Build history of the part. All positions in model axes, mm. Face numbers are marked on the shaded views. Round coordinates to 2 decimals unless told otherwise and drop trailing zeros. Loops run counter-clockwise (first coordinate to the right, second up) from the corner with the lowest first, then second, coordinate; pieces in that order, holes last. Notation, with made-up numbers: (89, -30) - (137, -30) arc R25 ccw to (137, -7) - close; hole circle Ø4 at (-35.75, 56). An arc over 180 degrees is marked (long way). Put each result on its own line as item: value. Start each with the question number.
from build123d import *

# Parameters (mm, degrees)
SKETCH2_W                                       = 20
SKETCH2_H                                       = 44
BOSS_EXTRUDE2_DEPTH                             = 0.5
SKETCH4_R                                       = 3.5
BOSS_EXTRUDE3_DEPTH                             = 8
CSK_FOR_M3_FLAT_HEAD_MACHINE_SCREW1_D           = 3.2
CSK_FOR_M3_FLAT_HEAD_MACHINE_SCREW1_DEPTH       = 13.03862301
CSK_FOR_M3_FLAT_HEAD_MACHINE_SCREW1_CSINK_D     = 6.3
CSK_FOR_M3_FLAT_HEAD_MACHINE_SCREW1_CSINK_ANGLE = 90
CSK_FOR_M3_FLAT_HEAD_MACHINE_SCREW1_TIP         = 0.96137699


with BuildPart() as part:
    # Sketch2 → Boss-Extrude2 (new body)
    with BuildSketch(Plane(origin=(0, 0, 0), x_dir=(1, 0, 0), z_dir=(0, 1, 0))):
        with Locations((10, 22)):
            Rectangle(SKETCH2_W, SKETCH2_H)
    extrude(amount=BOSS_EXTRUDE2_DEPTH)

    # Sketch4 → Boss-Extrude3 (add)
    with BuildSketch(Plane(origin=(0, 0, 0), x_dir=(1, 0, 0), z_dir=(0, 1, 0))):
        with Locations(Location((20, 44, 0), (0, 0, 270))):
            Circle(SKETCH4_R)
        with Locations(Location((0, 44, 0), (0, 0, 90))):
            Circle(SKETCH4_R)
        with Locations(Location((20, 0, 0), (0, 0, 90))):
            Circle(SKETCH4_R)
        with Locations(Location((0, 0, 0), (0, 0, 90))):
            Circle(SKETCH4_R)
    extrude(amount=BOSS_EXTRUDE3_DEPTH)

    # CSK for M3 Flat Head Machine Screw1
    with Locations(Plane(origin=(0, 8, 0), x_dir=(1, 0, 0), z_dir=(0, 1, 0))):
        with Locations((20, 44), (0, 44), (0, 0), (20, 0)):
            CounterSinkHole(CSK_FOR_M3_FLAT_HEAD_MACHINE_SCREW1_D / 2, CSK_FOR_M3_FLAT_HEAD_MACHINE_SCREW1_CSINK_D / 2, depth=CSK_FOR_M3_FLAT_HEAD_MACHINE_SCREW1_DEPTH, counter_sink_angle=CSK_FOR_M3_FLAT_HEAD_MACHINE_SCREW1_CSINK_ANGLE)
            with Locations((0, 0, -(CSK_FOR_M3_FLAT_HEAD_MACHINE_SCREW1_DEPTH + CSK_FOR_M3_FLAT_HEAD_MACHINE_SCREW1_TIP / 2))):  # 118° drill point
                Cone(0, CSK_FOR_M3_FLAT_HEAD_MACHINE_SCREW1_D / 2, CSK_FOR_M3_FLAT_HEAD_MACHINE_SCREW1_TIP, mode=Mode.SUBTRACT)


solid = part.part
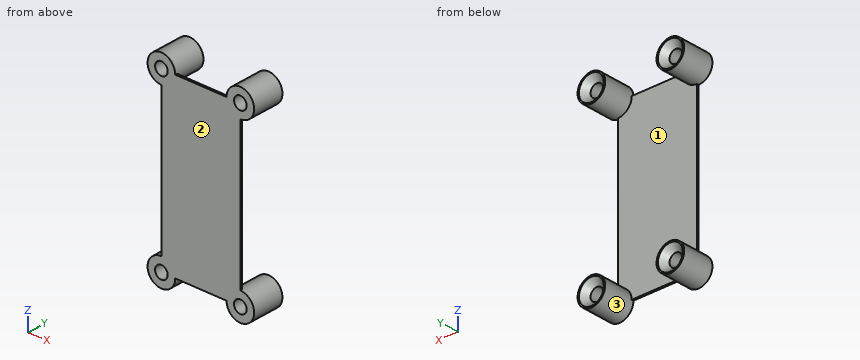
Item 1: Drop flat-ended pins along their axis: pin 1 Ø1.9 at (x, z) = (0, -44) entering from -Y; pin 2 Ø1 at (x, y) = (17, 6.5) entering from -Z; pin 3 Ø5 at (x, z) = (20, 0) entering from +Y; pin 4 Ø4 at (x, z) = (12, -8.5) entering from +Y. Give the stop position or say it passes through.
Item 2: Slice it at A-A (y = 4). Give the cut face in (x, z), plus the area to 3 significant figures.
Item 3: Drill centre lines: probe 1 along Z at (x, y) = (20, 1.5); probe 2 along X at (y, z) = (4.75, -1); probe 3 along X at (y, z) = (7.75, -2). Where is each one in solid material? Low to high. Write a range as [from, to].
Item 4: Slice it at B-B (x = 8.5). Give the cut face in (y, z), plus the area to 3 significant figures.
Item 5: Two-plate mould, pull along Z, no slides. Class the marked faces 1, 2 and 3: pulls with the +Z half, pulls with the -Z half, needs draft (parallel to the pull), parting line crosses it, or undercut.
Item 6: Slice it at C-C (x = 0.75). Give the number of separate pieces and of enclosed holes in the cut face, plus the area to 3 significant figures.
Item 7: Slice it at D-D (z = -5.5). Give the cut face in (x, y).
Computed values:
1. pin 1: passes through
1. pin 2: stops at z = -46.45
1. pin 3: stops at y = 7.35
1. pin 4: stops at y = 0.5
2. outline: circle Ø7 at (0, -44); circle Ø7 at (0, 0); circle Ø7 at (20, -44); circle Ø7 at (20, 0); hole circle Ø3.2 at (0, -44); hole circle Ø3.2 at (0, 0); hole circle Ø3.2 at (20, -44); hole circle Ø3.2 at (20, 0)
2. area: 122 mm^2
3. probe 1: z = [-47.5, -45.6], [-42.4, -40.5], [-3.5, -1.6], [1.6, 3.5]
3. probe 2: x = [-3.35, -1.25], [1.25, 3.35], [16.65, 18.75], [21.25, 23.35]
3. probe 3: x = [-2.87, -2.1], [2.1, 2.87], [17.13, 17.9], [22.1, 22.87]
4. outline: (0, -44) - (0.5, -44) - (0.5, 0) - (0, 0) - close
4. area: 22.0 mm^2
5. face 1: undercut
5. face 2: needs draft
5. face 3: undercut
6. separate pieces: 3
6. enclosed holes: 0
6. area: 77.6 mm^2
7. outline: (0, 0) - (20, 0) - (20, 0.5) - (0, 0.5) - close
